Could you check a few things on this model? Use its own coordinates, in mm. Round coordinates to 2 decimals unless told otherwise and drop trailing zeros. Write each loop counter-clockwise with the first axis right and the second up, starting at its lowest first coordinate (ties: lowest second). Pieces come first, ordered by that corner, then holes. Notation, with made-up numbers: (-11.75, 44) - (0.25, 44) arc R21 cw to (0.25, 50) - close; hole circle Ø3 at (87, 25.5). An arc over 180 degrees is marked (long way). Put each result on its own line as item: value.
from build123d import *

# Parameters (mm, degrees)
SKETCH1_R           = 2
BOSS_EXTRUDE1_DEPTH = 250


with BuildPart() as part:
    # Sketch1 → Boss-Extrude1 (new body)
    with BuildSketch(Plane(origin=(0, 0, 0), x_dir=(1, 0, 0), z_dir=(0, 1, 0))):
        with Locations(Location((0, 0, 0), (0, 0, 270))):
            Circle(SKETCH1_R)
    extrude(amount=BOSS_EXTRUDE1_DEPTH)

    # Sketch2 → Revolve1 (revolve)
    with BuildSketch(Plane.XY):
        with BuildLine():
            Line((4.25, 254.7141137), (5.120826884, 254.7141137))
            ThreePointArc((5.120826884, 254.7141137), (3.620971415, 251.093142285), (0, 249.593286816))
            Line((0, 249.593286816), (0, 250.4641137))
            ThreePointArc((0, 250.4641137), (3.00520382, 251.70890988), (4.25, 254.7141137))
        make_face()
    revolve1 = revolve(axis=Axis((0, 250.4641137, 0), (0, -1, 0)))

    # Mirror1: Revolve1 across plane
    add(revolve1.mirror(Plane(origin=(0, 125, 0), x_dir=(0, 0, 1), z_dir=(0, -1, 0))))


solid = part.part
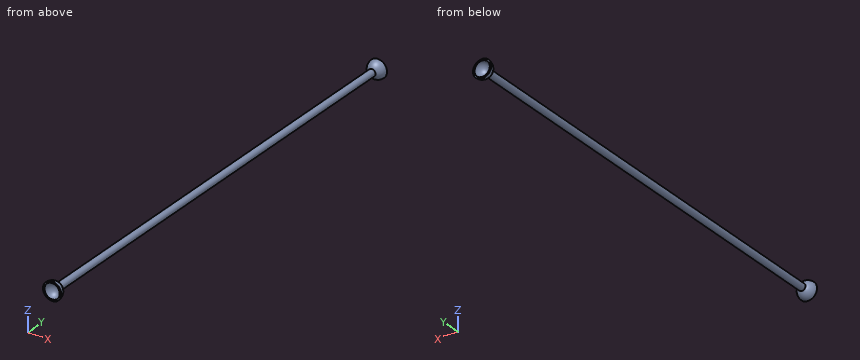
(1) Imagine slicing it at B-B, the plane z = 0. List the corners of the cut face in (x, y) for me, then the cut area to 3 significant figures.
Values found:
outline: (-5.12, -4.71) - (-4.25, -4.71) arc R4.25 cw to (4.25, -4.71) - (5.12, -4.71) arc R5.12 ccw to (2, 0) - (2, 250) arc R5.12 ccw to (5.12, 254.71) - (4.25, 254.71) arc R4.25 cw to (-4.25, 254.71) - (-5.12, 254.71) arc R5.12 ccw to (-2, 250) - (-2, 0) arc R5.12 ccw to start
area: 1,020 mm^2
(2) Please list where these lines run through material, in increasing order: probe 1 along Y at (x, z) = (-2, 2); probe 2 along Y at (x, z) = (-0.25, -0.25); probe 3 along Y at (x, z) = (0, -3.5). Write a range as from..to.
Values found:
probe 1: y = -1.54..-0.45, 250.45..251.54
probe 2: y = -0.48..250.48
probe 3: y = -2.3..-0.98, 250.98..252.3
(3) Imagine slicing it at C-C, the plane y = 52.5. List the corners of the cut face in (x, z) for me, then the cut area to 3 significant figures.
Values found:
outline: circle Ø4 at (0, 0)
area: 12.6 mm^2
(4) I'm going to push flat-ended pins straight in: pin 1 (1.5 mm diameter, centred on x = 2, z = -1, fed in from +Y); pin 2 (5 mm diameter, centred on x = 2.5, y = 186, fed in from -Z); pin 3 (2 mm diameter, centred on x = -2, y = 56.5, fed in from -Z); pin 4 (3 mm diameter, centred on x = 4, y = 203, fed in from +Z). Where does each tip first touch, or does it pass through?
Values found:
pin 1: stops at y = 251.69
pin 2: stops at z = -2
pin 3: stops at z = -1.73
pin 4: passes through
(5) Imagine slicing it at A-A, the plane x = 0. List the corners of the cut face in (y, z) for me.
Values found:
outline: (-4.71, -5.12) arc R5.12 ccw to (0, -2) - (250, -2) arc R5.12 ccw to (254.71, -5.12) - (254.71, -4.25) arc R4.25 cw to (254.71, 4.25) - (254.71, 5.12) arc R5.12 ccw to (250, 2) - (0, 2) arc R5.12 ccw to (-4.71, 5.12) - (-4.71, 4.25) arc R4.25 cw to (-4.71, -4.25) - close
